The model under review builds one solid part; all positions refer to its coordinate system, in mm. A direction names the side the tool comes from. Coordinates: 2 decimals unless noted, no trailing zeros. Write each loop counter-clockwise with the first axis right and the second up, starting at its lowest first coordinate (ties: lowest second). Pieces come first, ordered by that corner, then holes. Notation, with made-up numbers: (-27.75, 40) - (20.25, 40) arc R27 cw to (20.25, 64) - close; hole circle Ø4 at (35.25, 35). An arc over 180 degrees is marked (long way). Put each result on its own line as item: value. Start each with the question number.
Item 1: To check wall thickness, follow L1, parallel to Y at x = 9, z = -0.95; L2, parallel to X at y = 0.85, z = 0.5; L3, parallel to Z at x = 31, y = -0.15. State the ranges of each line that lie inside material, in increasing order. Write a range as [from, to].
Item 2: For pin 1 (0.6 mm diameter, centred on x = -1, z = 0, fed in from -Y), flat-tipped, find the tip position at first contact; note if it passes through.
Item 3: Mouldability with a two-part tool opening along Y and no side actions: class faces 4 (the face through (17.15, -1.5, -0.07)), 5 (the face through (0, 0.1, 0)), 6 (the face through (35, 0, 0)), 7 (the face through (-1.09, -0.49, 0.87)) as pulls with the +Y half, pulls with the -Y half, needs draft (parallel to the pull), parting line crosses it, or undercut.
Item 4: Consider section A-A on x = 17. Give the boundary of the cut face in (y, z).
Item 5: Machinability: for faces 1 (the face through (0, 0, -2)), 2 (the face through (-0.193, -2.262, 1.734)), 3 (the face through (-1, -1, 0)), which of the approach directions +Z, -Z, +X, -X, +Y, -Y give a long, thin tool a straight path to every point of the face, cutting with its end or side? Answer none if there is none.
Autodesk Inventor part; units mm, degrees
ref_plane "Work Plane1" through (30, 0, 0) normal (0, -0.5, 0.866) x (1, 0, 0)
ref_plane "YZ Plane" through (0, 0, 0) normal (1, 0, 0) x (0, 1, 0)
ref_plane "XZ Plane" through (0, 0, 0) normal (0, 1, 0) x (-1, 0, 0)
sketch "Sketch1" plane through (0, 0, 0) normal (0, 0, 1) x (1, 0, 0)
  line L0 (0.0567, 0) -> (35, 0)
  line L1 (35, 0) -> (35, 1.5)
  line L2 (35, 1.5) -> (1, 1.5)
  line L3 (1, 1.5) -> (0.6933, 1.5)
  line L4 (0.6933, 1.5) -> (0, 1.5)
  line L5 (0, 1.5) -> (0, 2.85)
  line L6 (0, 2.85) -> (-1.65, 2.85)
  line L7 (-1.65, 2.85) -> (-1.65, 1.1547)
  line L8 (-1.65, 1.1547) -> (-0.61, 1.1547)
  line L9 (-0.61, 1.1547) -> (0.0567, 0)
  line L10 (-8.98, 0) -> (42.33, 0)
  line L11 (0, -0.57) -> (0, 3.42)
  line L12 (1, 1.5) -> (0, 1.5) construction
  dimension "d0" = 34
  dimension "d1" = 0.3067
  dimension "d2" = 1.65
  dimension "d3" = 1.04
  dimension "d4" = 60
  dimension "d5" = 3
  dimension "d6" = 3
  dimension "d7" = 2.3094
  dimension "d8" = 5.7
  dimension "d19" = 35
revolve "Body" add sketch "Sketch1" angle 360 about axis through (0.0567, 0, 0) along (1, 0, 0) contours L9 L11 L4 L3 L2 L1 L0 | L9 L8 L7 L6 L5 L11
sketch "Sketch2" plane through (-1.65, 0, 0) normal (-1, 0, 0) x (0, 0, 1)
  circle A0 centre (0, 0) radius 1.1547
  line L0 (0, -3.99) -> (0, 3.99)
  line L1 (-3.99, 0) -> (3.99, 0)
  line L2 (1.1547, 0) -> (0.5774, -1)
  line L3 (0.5774, -1) -> (-0.5774, -1)
  line L4 (-0.5774, -1) -> (-1.1547, 0)
  line L5 (-1.1547, 0) -> (-0.5774, 1)
  line L6 (-0.5774, 1) -> (0.5774, 1)
  line L7 (0.5774, 1) -> (1.1547, 0)
extrude "Slot" add sketch "Sketch2" against normal up to next contours L7 A0 | A0 L2 | L6 L0 A0 | A0 L0 L3 | L0 L6 A0 | A0 L3 L0 | L4 A0 | A0 L5
fillet "Fillet1" radius 1.27 1 edges at (-1.65, -2.85, 0)
thread "Thread"
chamfer "Chamfer1" distance 0.3067 distance2 0.3067 1 edges at (35, -1.5, 0) measured on face at (35, -0.8773, -0.3972)
fillet "Fillet2" radius 0.1 1 edges at (0, -1.5, 0)
ref_plane "Work Plane1" through (30, 0, 0) normal (0, -0.5, 0.866) x (1, 0, 0)
equation "\"d16\" = RR"
equation "\"d12\" = GEL"
equation "\"d14\" = -0.5 * SPD + 0.5 * GD"
equation "\"d15\" = GUL"
equation "\"d29\" = R"
equation "\"d0\" = GEL"
equation "\"d1\" = GAL"
equation "\"d2\" = KOH"
equation "\"d3\" = INTI"
equation "\"d5\" = GD"
equation "\"d6\" = BDM"
equation "\"d7\" = 1.1547 * SW"
equation "\"d8\" = KOD"
equation "\"d19\" = NLG"
equation "\"GD\" = NND"
equation "\"NLG\" = 35"
equation "\"GEL\" = 34"
equation "\"KOD\" = 5.7"
equation "\"KOH\" = 1.65"
equation "\"INTI\" = 1.04"
equation "\"GAL\" = 0.61345 * PTC"
equation "\"GUL\" = 0.61345 * PTC"
equation "\"BDM\" = NND"
equation "\"SW\" = 2"
equation "\"RR\" = 1.27"
equation "\"SPD\" = 2.38655"
equation "\"d28\" = R"
equation "\"R\" = 0.1"
equation "\"TOA\" = 30deg"
equation "\"THREADDIA\" = 3"
equation "\"KOD1\" = KOD - 2 * RR"
equation "\"PTC\" = 0.5"
equation "\"NND\" = 3"
equation "\"E0\" = 1.155 * SW"
equation "\"GD1\" = THREADDIA - 1.2269 * PTC"
properties part number "ANSI B18.3.4M - M3 x 0.5 x 35, FHSBHCSM" material "Steel, Mild"
Report:
1. L1: [-1.16, 1.16]
1. L2: [-0.51, 35]
1. L3: [-1.49, 1.49]
2. pin 1: y = -2.81
3. face 4: parting line crosses it
3. face 5: undercut
3. face 6: needs draft
3. face 7: undercut
4. outline: circle Ø3 at (0, 0)
5. face 1: +X
5. face 2: +X, -X
5. face 3: -X
